For this review, take the finished solid that the model builds, in its own axes (mm). Give positions to 0.01 mm unless a question says otherwise; leave off trailing zeros. Loops run counter-clockwise (first coordinate to the right, second up) from the corner with the lowest first, then second, coordinate; pieces in that order, holes last.
```python
from build123d import *

# Parameters (mm, degrees)
SKETCH1_W           = 250
SKETCH1_H           = 42
SKETCH1_W_2         = 12.7
SKETCH1_H_2         = 15
BOSS_EXTRUDE1_DEPTH = 6.35
SKETCH2_W           = 6.35
SKETCH2_H           = 15
CUT_EXTRUDE1_DEPTH  = 140.436768824
LPATTERN1_COUNT     = 3
LPATTERN1_PITCH     = 60
SKETCH3_W           = 65
SKETCH3_H           = 8
CUT_EXTRUDE2_DEPTH  = 140.436768824
SKETCH4_W           = 20
SKETCH4_H           = 6.35
BOSS_EXTRUDE2_DEPTH = 6.35


with BuildPart() as part:
    # Sketch1 → Boss-Extrude1 (new body)
    with BuildSketch(Plane(origin=(0, 0, 0), x_dir=(0, 0, -1), z_dir=(1, 0, 0))):
        Rectangle(SKETCH1_W, SKETCH1_H)
        with Locations((-131.35, 0)):
            Rectangle(SKETCH1_W_2, SKETCH1_H_2)
    extrude(amount=BOSS_EXTRUDE1_DEPTH)

    # Sketch2 → Cut-Extrude1 (cut, through all)
    with BuildSketch(Plane(origin=(6.35, 0, 0), x_dir=(0, 0, -1), z_dir=(1, 0, 0))):
        with Locations((-72.825, 0)):
            Rectangle(SKETCH2_W, SKETCH2_H)
    cut_extrude1 = extrude(amount=-CUT_EXTRUDE1_DEPTH, mode=Mode.SUBTRACT)

    # LPattern1: Cut-Extrude1 ×3
    with Locations(*[(0, 0, -i * LPATTERN1_PITCH) for i in range(1, LPATTERN1_COUNT)]):
        add(cut_extrude1, mode=Mode.SUBTRACT)

    # Sketch3 → Cut-Extrude2 (cut, through all)
    with BuildSketch(Plane(origin=(6.35, 0, 0), x_dir=(0, 0, -1), z_dir=(1, 0, 0))):
        with Locations((92.5, 0)):
            Rectangle(SKETCH3_W, SKETCH3_H)
    extrude(amount=-CUT_EXTRUDE2_DEPTH, mode=Mode.SUBTRACT)

    # Sketch4 → Boss-Extrude2 (add)
    with BuildSketch(Plane(origin=(6.35, 0, 0), x_dir=(0, 0, -1), z_dir=(1, 0, 0))):
        with Locations((-42.825, 24.175)):
            Rectangle(SKETCH4_W, SKETCH4_H)
        with Locations((17.175, 24.175)):
            Rectangle(SKETCH4_W, SKETCH4_H)
    boss_extrude2 = extrude(amount=-BOSS_EXTRUDE2_DEPTH)

    # Mirror1: Boss-Extrude2 across plane
    add(boss_extrude2.mirror(Plane.ZX))


solid = part.part
```
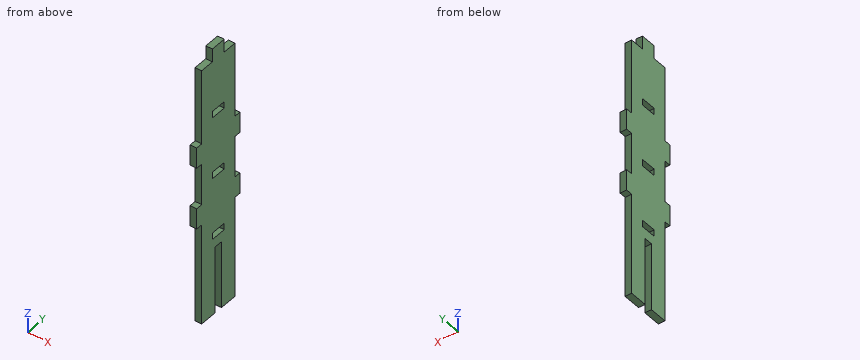
Q1. For probe 1 along Z at (x, y) = (5.5, 5.5); probe 2 along Z at (x, y) = (1, -2); probe 3 along Z at (x, y) = (0.75, 23.5) (3 decimals), list the stretches that pass through material, from the lowest coordinate up.
Answers:
probe 1: z = -125 to -50.35, -44 to 9.65, 16 to 69.65, 76 to 137.7
probe 2: z = -60 to -50.35, -44 to 9.65, 16 to 69.65, 76 to 137.7
probe 3: z = -27.175 to -7.175, 32.825 to 52.825
Q2. Consider section A-A on y = -1. Give the boundary of the cut face in (x, z).
Answers:
outline: (0, -60) - (6.35, -60) - (6.35, -50.35) - (0, -50.35) - close; (0, -44) - (6.35, -44) - (6.35, 9.65) - (0, 9.65) - close; (0, 16) - (6.35, 16) - (6.35, 69.65) - (0, 69.65) - close; (0, 76) - (6.35, 76) - (6.35, 137.7) - (0, 137.7) - close
Q3. Consider section C-C on y = 23.5. Give the boundary of the cut face in (x, z) (3 decimals), plus the area to 3 significant figures.
Answers:
outline: (0, -27.175) - (6.35, -27.175) - (6.35, -7.175) - (0, -7.175) - close; (0, 32.825) - (6.35, 32.825) - (6.35, 52.825) - (0, 52.825) - close
area: 254 mm2
Q4. Consider section D-D on x = 4.25. Count the separate pieces of the cut face and the enclosed holes in it, plus the area to 3 significant figures.
Answers:
separate pieces: 1
enclosed holes: 3
area: 10,400 mm2
Q5. Consider section B-B on z = -86. Give the boundary of the cut face in (x, y), plus the area to 3 significant figures.
Answers:
outline: (0, -21) - (6.35, -21) - (6.35, -4) - (0, -4) - close; (0, 4) - (6.35, 4) - (6.35, 21) - (0, 21) - close
area: 216 mm2
Q6. For pin 1 Ø3 at (x, z) = (3, 11.5) entering from -Y; pin 2 Ø1.9 at (x, z) = (2, 71.5) entering from +Y; pin 3 Ø1.9 at (x, y) = (1.5, 25) entering from +Z (3 decimals), all flat-tipped, find the tip position at first contact; note any pin that passes through.
Answers:
pin 1: stops at y = -21
pin 2: stops at y = 21
pin 3: stops at z = 52.825
